from build123d import *

# Parameters (mm, degrees)
BOSS_EXTRUDE1_DEPTH = 34.5
SKETCH1_4_R         = 14
BOSS_EXTRUDE2_DEPTH = 19
BOSS_EXTRUDE3_DEPTH = 13


with BuildPart() as part:
    # Sketch1 → Boss-Extrude1 (new body)
    with BuildSketch(Plane(origin=(0, 0, 0), x_dir=(1, 0, 0), z_dir=(0, 1, 0))):
        with BuildLine():
            Line((-4.053189053, -10.226028173), (-4.050853741, -10.220136277))
            Line((-4.050853741, -10.220136277), (-4.050853741, -2.498244783))
            Line((-4.050853741, -2.498244783), (-10.712551829, -2.498244783))
            ThreePointArc((-10.712551829, -2.498244783), (-8.332852752, -7.180777027), (-4.053189053, -10.226028173))
        make_face()
        with BuildLine():
            Line((-10.712551829, -2.498244783), (-4.050853741, -2.498244783))
            Line((-4.050853741, -2.498244783), (-4.050853741, 2.501755217))
            Line((-4.050853741, 2.501755217), (-10.711732564, 2.501755217))
            ThreePointArc((-10.711732564, 2.501755217), (-10.999999566, 0.001802383), (-10.712551829, -2.498244783))
        make_face()
        with BuildLine():
            Line((-10.711732564, 2.501755217), (-4.050853741, 2.501755217))
            Line((-4.050853741, 2.501755217), (-4.050853741, 10.226953489))
            ThreePointArc((-4.050853741, 10.226953489), (-8.33085594, 7.183093554), (-10.711732564, 2.501755217))
        make_face()
        with BuildLine():
            Line((4.050853741, 10.226953489), (4.050853741, 2.5))
            Line((4.050853741, 2.5), (10.712142348, 2.5))
            ThreePointArc((10.712142348, 2.5), (8.331444409, 7.182410999), (4.050853741, 10.226953489))
        make_face()
        with BuildLine():
            Line((4.050853741, 2.5), (4.050853741, -2.498244783))
            Line((4.050853741, -2.498244783), (10.712551829, -2.498244783))
            ThreePointArc((10.712551829, -2.498244783), (10.927901462, -1.257363639), (10.999999713, 0))
            ThreePointArc((10.999999713, 0), (10.927798416, 1.258258902), (10.712142348, 2.5))
            Line((10.712142348, 2.5), (4.050853741, 2.5))
        make_face()
        with BuildLine():
            Line((4.050853741, -2.498244783), (4.050853741, -10.226953489))
            ThreePointArc((4.050853741, -10.226953489), (8.332032799, -7.181728421), (10.712551829, -2.498244783))
            Line((10.712551829, -2.498244783), (4.050853741, -2.498244783))
        make_face()
    extrude(amount=BOSS_EXTRUDE1_DEPTH)

    # Sketch1_4 → Boss-Extrude2 (add)
    with BuildSketch(Plane(origin=(0, 0, 0), x_dir=(1, 0, 0), z_dir=(0, 1, 0))):
        with Locations(Location((0, 0, 0), (0, 0, 270))):
            Circle(SKETCH1_4_R)
        with BuildLine():
            Line((4.050853741, -10.226953489), (4.050853741, 2.5))
            Line((4.050853741, 2.5), (4.050853741, 10.226953489))
            ThreePointArc((4.050853741, 10.226953489), (10.999999713, 0), (4.050853741, -10.226953489))
        make_face(mode=Mode.SUBTRACT)
        with BuildLine():
            Line((-4.050853741, -10.220136277), (-4.050853741, -10.226953489))
            ThreePointArc((-4.050853741, -10.226953489), (-10.999999713, 0), (-4.050853741, 10.226953489))
            Line((-4.050853741, 10.226953489), (-4.050853741, 2.501755217))
            Line((-4.050853741, 2.501755217), (-4.050853741, -10.220136277))
        make_face(mode=Mode.SUBTRACT)
    extrude(amount=BOSS_EXTRUDE2_DEPTH)

    # Sketch1_5 → Boss-Extrude3 (add)
    with BuildSketch(Plane(origin=(0, 0, 0), x_dir=(1, 0, 0), z_dir=(0, 1, 0))):
        with BuildLine():
            Line((-16, -2.498244783), (-13.77529575, -2.498244783))
            ThreePointArc((-13.77529575, -2.498244783), (-13.999999886, 0.001783889), (-13.774658647, 2.501755217))
            Line((-13.774658647, 2.501755217), (-16, 2.501755217))
            Line((-16, 2.501755217), (-16, -2.498244783))
        make_face()
        with BuildLine():
            ThreePointArc((14, 0), (13.943710778, -1.254164961), (13.77529575, -2.498244783))
            Line((13.77529575, -2.498244783), (15.995322261, -2.498244783))
            Line((15.995322261, -2.498244783), (15.995322261, 2.5))
            Line((15.995322261, 2.5), (13.774977314, 2.5))
            ThreePointArc((13.774977314, 2.5), (13.943630847, 1.255053307), (14, 0))
        make_face()
    extrude(amount=BOSS_EXTRUDE3_DEPTH)


solid = part.part
Model file for the job. Use its own axes, mm. A direction names the side the tool comes from. Coordinates: 2 decimals unless noted, no trailing zeros. Order: outer loops, then holes, each group sorted by start corner. A loop starts at its lowest first (then second) coordinate and runs counter-clockwise, first axis right, second up. Notation, with made-up numbers: M 82,43 L 141,43 A35 ccw 141,81 Z; hole C 80.25,13.5 d7. An arc over 180 degrees is marked long. Return JSON: item names as keys, results as strings.
1. Pull direction X, two halves, no side cores. Call faces 4 (the face through (0, 19, 0)), 5 (the face through (0, 0, 0)), 6 (the face through (-4.051, 27, 0)), 7 (the face through (-12.4, 9.4, 6.5)): +X half, -X half, draft (parallel to the pull), parting line (faces both ways), or undercut.
Ans:
{"face 4": "undercut", "face 5": "draft", "face 6": "undercut", "face 7": "parting line"}
2. Flat gauge pins, fed straight in: pin 1 (2.5 mm diameter, centred on x = 15.5, z = 0, fed in from +Y); pin 2 (1.5 mm diameter, centred on x = 7, y = 23.5, fed in from -Z); pin 3 (4.5 mm diameter, centred on y = 27, z = 1, fed in from +X). Where does each tip first touch, or does it go through?
Ans:
{"pin 1": "y = 13", "pin 2": "z = -9.05", "pin 3": "x = 11"}
3. Drill centre lines: probe 1 along Y at (x, z) = (-12.5, -1); probe 2 along X at (y, z) = (30.5, -2); probe 3 along X at (y, z) = (9, 4.5). Where is each one in solid material? Low to high.
Ans:
{"probe 1": "0 to 19", "probe 2": "-10.82 to -4.05, 4.05 to 10.82", "probe 3": "-13.26 to 13.26"}
4. Saw through at D-D (x = 0). Give the cut face in (y, z).
Ans:
{"outline": "M 0,-14 L 19,-14 L 19,14 L 0,14 Z"}
5. Tool access for faces 1 (the face through (-15, 6, -2.502)), 2 (the face through (15, 6, -2.5)), 3 (the face through (4.051, 27, 0)): list every direction of +Z, -Z, +X, -X, +Y, -Y with a clear straight run to the whole face (end or side of a thin tool).
Ans:
{"face 1": "-Z, -X, +Y, -Y", "face 2": "-Z, +X, +Y, -Y", "face 3": "+Z, -Z, +Y"}
6. Saw through at C-C (z = 6.5). Give the cut face in (x, y), and give its area (3 significant figures).
Ans:
{"outline": "M -12.4,0 L 12.4,0 L 12.4,19 L 8.87,19 L 8.87,34.5 L 4.05,34.5 L 4.05,19 L -4.05,19 L -4.05,34.5 L -8.87,34.5 L -8.87,19 L -12.4,19 Z", "area": "621 mm^2"}
